Design review of the part shown in the three views and the two pictorial views. Dimensions are in mm from the part's minimum x, y and z. A direction names the side the tool comes from. Give positions to 0.01 mm unless a question says otherwise; leave off trailing zeros. Write each loop counter-clockwise with the first axis right and the second up, starting at its lowest first coordinate (ties: lowest second). Pieces come first, ordered by that corner, then holes. Notation, with made-up numbers: M 37,-5.75 L 77,-5.75 A23 cw 77,24.25 Z; hole C 15,-33.5 d7. An arc over 180 degrees is marked long. Use one line per item in the form item = value. Start each with the question number.
Q1. Consider section D-D on x = 2.75. Write out the cut boundary in (y, z).
Q2. Clearance check with flat-ended pins moving along their axes: pin 1 Ø0.5 at (y, z) = (0.5, 8) entering from -X; pin 2 Ø0.8 at (y, z) = (11.5, 7) entering from +X. State where each tip first meets the part, or that it passes through.
Q3. Consider section C-C on y = 3.5. Write out the cut boundary in (x, z).
Q4. For probe 1 along Z at (x, y) = (4.5, 6); probe 2 along Z at (x, y) = (6.5, 7); probe 3 along X at (y, z) = (7.75, 10.75), list the stretches that pass through material, from the lowest coordinate up. Write a range as [from, to].
Q5. Consider section B-B on x = 5.75. Write out the cut boundary in (y, z), and give its area (3 significant figures).
Q6. Tool access review of the marked faces 1 and 2: name each direction out of +Z, -Z, +X, -X, +Y, -Y from which nothing blocks a thin tool from reaching the whole face with its end or side.
Q7. Mouldability with a two-part tool opening along Y and no side actions: class the marked faces 3 and 4 as released by +Y, released by -Y, zero draft, split by the parting line, or undercut.
Q8. Consider section A-A on y = 6. Write out the cut boundary in (x, z).
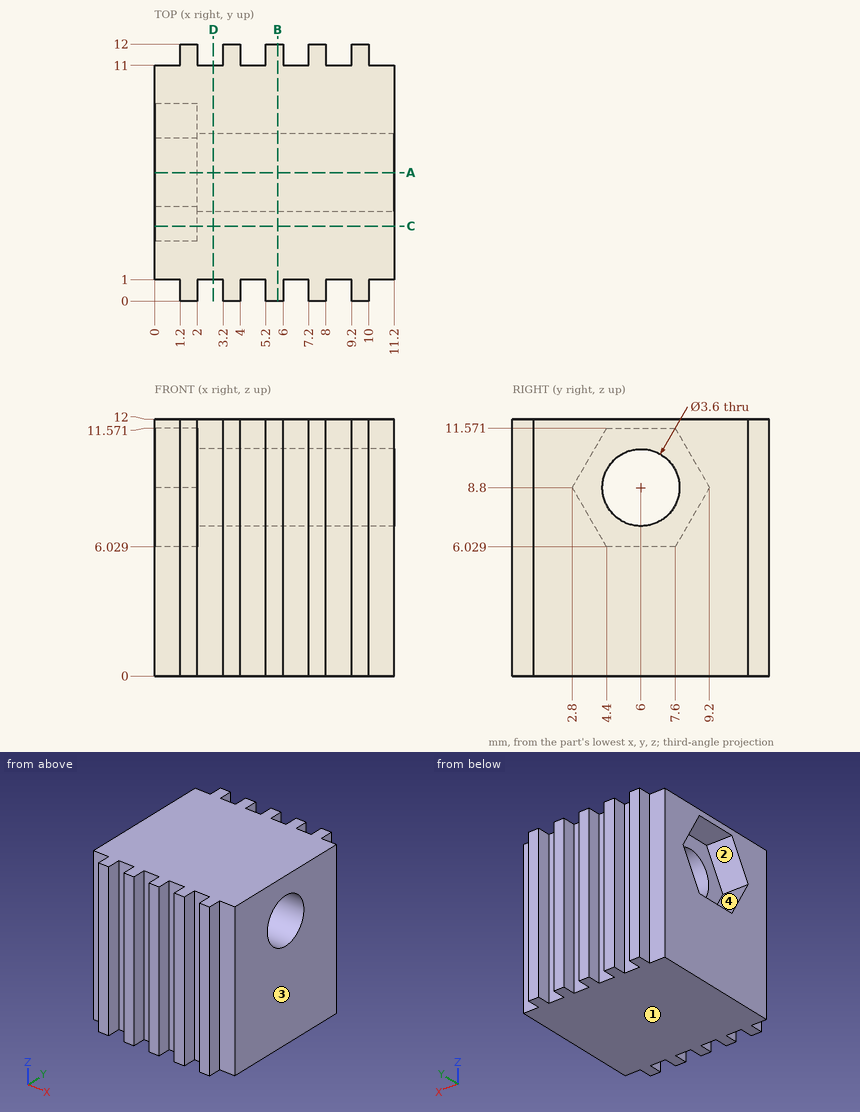
Working result:
q1.outline = M 1,0 L 11,0 L 11,12 L 1,12 Z; hole C 6,8.8 d3.6
q2.pin_1 = 1.2
q2.pin_2 = 10
q3.outline = M 0,0 L 11.2,0 L 11.2,12 L 0,12 L 0,10.01 L 2,10.01 L 2,7.59 L 0,7.59 Z
q4.probe_1 = [0, 7], [10.6, 12]
q4.probe_2 = [0, 7.3], [10.3, 12]
q4.probe_3 = [2, 11.2]
q5.outline = M 0,0 L 12,0 L 12,12 L 0,12 Z; hole C 6,8.8 d3.6
q5.area = 134 mm²
q6.face_1 = -Z, +X, -X, +Y, -Y
q6.face_2 = -X
q7.face_3 = zero draft
q7.face_4 = undercut
q8.outline = M 0,0 L 11.2,0 L 11.2,7 L 2,7 L 2,6.03 L 0,6.03 Z; M 0,11.57 L 2,11.57 L 2,10.6 L 11.2,10.6 L 11.2,12 L 0,12 Z
